Work out the finished part from the listing and answer in its coordinate system (mm). Round coordinates to 2 decimals unless told otherwise and drop trailing zeros. Use a Markdown table: item, result. Add a question column.
Item 1: Find the intervals of material crossed by L1, parallel to Y at x = 25, z = 0.2; L2, parallel to Y at x = -1, z = 0.1; L3, parallel to Y at x = 27.5, z = -0.1, in increasing order. Write a range as [from, to].
Item 2: A cutting plane is placed at A-A, the plane z = 0.1. Give the number of separate pieces and of enclosed holes in the cut face, plus the area to 3 significant figures.
Item 3: For a pull along Y with two mould halves and no side action, classify faces 1 (the cylindrical face through (25.08, -3.7, 0)), 2 (the flat face through (18, 1, -0.25)) as +Y half, -Y half, draft (parallel to the pull), parting line (faces both ways), or undercut.
from build123d import *

# Parameters (mm, degrees)
EXTRUDE_1_DEPTH     = 0.25
SKETCH_3_R          = 0.3
SKETCH_3_R_2        = 0.2
CUT_EXTRUDE_1_DEPTH = 0.25
EXTRUDE_2_DEPTH     = 0.25
FILLET_1_R          = 0.5
SKETCH_5_W          = 70.035704888
SKETCH_5_H          = 36.253776648
CUT_EXTRUDE_2_DEPTH = 0.25
FILLET_START        = -1
FILLET_2_DEPTH      = 2


with BuildPart() as part:
    # 草图2 → 凸台-拉伸1 (new, symmetric)
    with BuildSketch(Plane.XY):
        with BuildLine():
            ThreePointArc((94.3, -5.23), (94.279085645, -5.63954323), (94, -5.94))
            add(Edge.make_bspline(
                [(1.4, -2.38), (47.954561827, 5.976867864), (94, -5.94)],
                knots=[0, 0, 0, 1, 1, 1], degree=2))
            add(Edge.make_bspline(
                [(0, 0), (-4.123736473, -1.859487618), (1.4, -2.38)],
                knots=[0, 0, 0, 1, 1, 1], degree=2))
            add(Edge.make_bspline(
                [(0, 0), (47.273266317, 6.255778848), (94.3, -5.23)],
                knots=[0, 0, 0, 1, 1, 1], degree=2))
        make_face()
    extrude(amount=EXTRUDE_1_DEPTH, both=True)

    # 草图3 → 切除-拉伸1 (cut, symmetric)
    with BuildSketch(Plane.XY):
        with Locations((-1, -1.3)):
            Circle(SKETCH_3_R)
        with Locations((8.6, 0.4)):
            Circle(SKETCH_3_R)
        with Locations((25, 1.6)):
            Circle(SKETCH_3_R)
        with Locations((42.4, 1.5)):
            Circle(SKETCH_3_R)
        with Locations((68, -0.5)):
            Circle(SKETCH_3_R_2)
        with Locations((93.8, -5.5)):
            Circle(SKETCH_3_R_2)
    extrude(amount=CUT_EXTRUDE_1_DEPTH, both=True, mode=Mode.SUBTRACT)

    # 草图4 → 凸台-拉伸2 (add, symmetric)
    with BuildSketch(Plane.XY):
        with BuildLine():
            ThreePointArc((22.854587938, 0.396951856), (25.20918356, -4.692698154), (26.83283005, 0.675022949))
            add(Edge.make_bspline(
                [(22.854587938, 0.396951856), (24.844176287, 0.554595418), (26.83283005, 0.675022949)],
                knots=[0, 0, 0, 1, 1, 1], degree=2))
        make_face()
        with BuildLine():
            Line((24.7, 0.277371993), (24.7, -0.2))
            Line((24.7, -0.2), (25.3, -0.2))
            Line((25.3, -0.2), (25.3, 0.277371993))
            ThreePointArc((25.3, 0.277371993), (25, -3.7), (24.7, 0.277371993))
        make_face(mode=Mode.SUBTRACT)
    extrude(amount=EXTRUDE_2_DEPTH, both=True)

    # 圆角1
    fillet_1_edges = [part.edges().sort_by_distance(p)[0] for p in [
        (26.83283005, 0.675022949, -0.125),
        (22.854587938, 0.396951856, -0.125),
    ]]
    fillet(fillet_1_edges, radius=FILLET_1_R)

    # 草图5 → 切除-拉伸2 (cut, symmetric)
    with BuildSketch(Plane.XY):
        with Locations((79.017852444, -9.233575246)):
            Rectangle(SKETCH_5_W, SKETCH_5_H)
    extrude(amount=CUT_EXTRUDE_2_DEPTH, both=True, mode=Mode.SUBTRACT)

    # 圆角2: read off the stored shape, not the designer's step
    # 圆角2 outline → 圆角2 (cut)
    with BuildSketch(Plane.XY.offset(FILLET_START)):
        with BuildLine():
            add(Edge.make_bspline(
                [(44, 1.977919753), (43.768012094, 1.987811641), (43.536018221, 1.997274187)],
                knots=[0.534054584, 0.534054584, 0.534054584, 0.538973918, 0.538973918, 0.538973918], degree=2))
            add(Edge.make_bspline(
                [(43.536018221, 1.997274187), (43.770994303, 1.987690003), (44.000000033, 1.825022881), (44, 1.513981716)],
                knots=[0, 0, 0, 0, 0.492568205, 0.492568205, 0.492568205, 0.492568205], degree=3, weights=[1, 0.675356893, 0.510622658, 0.505797296]))
            Line((44, 1.513981716), (44, 1.977919753))
        make_face()
        with BuildLine():
            Line((44, 1.020922578), (44, 1.513981716))
            add(Edge.make_bspline(
                [(44, 1.513981716), (43.999999965, 1.187287005), (43.753387643, 1.02593813), (43.507593676, 1.030365965)],
                knots=[0.492568205, 0.492568205, 0.492568205, 0.492568205, 1, 1, 1, 1], degree=3, weights=[0.505797296, 0.500826325, 0.66556056, 1]))
            add(Edge.make_bspline(
                [(43.507593676, 1.030365965), (43.753804029, 1.025930629), (44, 1.020922578)],
                knots=[0.453363068, 0.453363068, 0.453363068, 0.458678061, 0.458678061, 0.458678061], degree=2))
        make_face()
    extrude(amount=FILLET_2_DEPTH, mode=Mode.SUBTRACT)


solid = part.part
Reported:
| question | item | result |
|---|---|---|
| 1 | L1 | [-4.7, -3.7], [-0.2, 1.3], [1.9, 2.07] |
| 1 | L2 | [-1.96, -1.6], [-1, -0.52] |
| 1 | L3 | [-3.36, -0.04], [0.52, 2.14] |
| 2 | separate pieces | 1 |
| 2 | enclosed holes | 5 |
| 2 | area | 89.4 mm² |
| 3 | face 1 | undercut |
| 3 | face 2 | draft |
